```python
from build123d import *

# Parameters (mm, degrees)
ESQUISSE1_R             = 15
BOSS_EXTRU_1_DEPTH      = 20
ESQUISSE3_R             = 13.5
ENL_V_MAT_EXTRU_2_DEPTH = 19
ESQUISSE4_R             = 12.5
BOSS_EXTRU_2_DEPTH      = 1
ESQUISSE5_R             = 11
ENL_V_MAT_EXTRU_3_DEPTH = 2


with BuildPart() as part:
    # Esquisse1 → Boss.-Extru.1 (new body)
    with BuildSketch(Plane.XY):
        Circle(ESQUISSE1_R)
    extrude(amount=BOSS_EXTRU_1_DEPTH)

    # Esquisse3 → Enlèv. mat.-Extru.2 (cut)
    with BuildSketch(Plane(origin=(0, 0, 0), x_dir=(-1, 0, 0), z_dir=(0, 0, -1))):
        Circle(ESQUISSE3_R)
    extrude(amount=-ENL_V_MAT_EXTRU_2_DEPTH, mode=Mode.SUBTRACT)

    # Esquisse4 → Boss.-Extru.2 (add)
    with BuildSketch(Plane.XY.offset(20)):
        Circle(ESQUISSE4_R)
    extrude(amount=BOSS_EXTRU_2_DEPTH)

    # Esquisse5 → Enlèv. mat.-Extru.3 (cut)
    with BuildSketch(Plane.XY.offset(21)):
        Circle(ESQUISSE5_R)
    extrude(amount=-ENL_V_MAT_EXTRU_3_DEPTH, mode=Mode.SUBTRACT)


solid = part.part
```
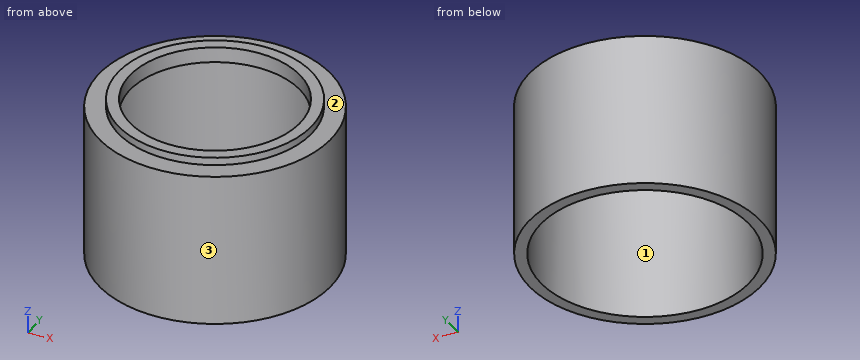
Check sheet for the modelled part. Datum: model origin and axes. Units: mm. Face numbers are marked on the shaded views. Coordinates: 2 decimals unless noted, no trailing zeros. Write each loop counter-clockwise with the first axis right and the second up, starting at its lowest first coordinate (ties: lowest second). Pieces come first, ordered by that corner, then holes. Notation, with made-up numbers: (55.5, -4) - (80.5, -4) arc R19 cw to (80.5, 23) - close; hole circle Ø10 at (-33.5, -27). An arc over 180 degrees is marked (long way). One line per question, with ' | ' between items.
Item 1: Thickness scan on line 1 (Y direction, x = 0, z = 20.1); line 2 (Y direction, x = 0, z = 11.75); line 3 (X direction, y = 4, z = 1.25). Record the ranges inside material, lowest first. Write a range as [from, to].
Determined:
line 1: y = [-12.5, -11], [11, 12.5] | line 2: y = [-15, -13.5], [13.5, 15] | line 3: x = [-14.46, -12.89], [12.89, 14.46]
Item 2: Gauge pin test, flat ends, axial feed: P1, Ø5, axis at x = 10.5, z = 17.5, coming from the +Y side; P2, Ø1, axis at x = -6.5, z = 15, coming from the +Y side; P3, Ø3, axis at x = -8, y = 5.5, coming from the +Z side; P4, Ø12, axis at y = -11, z = 18, coming from the -X side. Record the tip position at first contact, or that the pin passes through.
Determined:
P1: stops at y = 12.69 | P2: stops at y = 13.75 | P3: stops at z = 21 | P4: stops at x = -14.14
Item 3: Sectioned sample at C-C on z = 14.25. Record the boundary of the cut face in (x, y).
Determined:
outline: circle Ø30 at (0, 0); hole circle Ø27 at (0, 0)
Item 4: Sectioned sample at A-A on y = 0. Record the boundary of the cut face in (x, z), plus the area to 3 significant figures.
Determined:
outline: (-15, 0) - (-13.5, 0) - (-13.5, 19) - (-11, 19) - (-11, 21) - (-12.5, 21) - (-12.5, 20) - (-15, 20) - close; (11, 19) - (13.5, 19) - (13.5, 0) - (15, 0) - (15, 20) - (12.5, 20) - (12.5, 21) - (11, 21) - close | area: 68.0 mm2
Item 5: Mould release check, pull along Y, two halves, no side actions. Record for the marked faces 1, 2 and 3: pulls with the +Y half, pulls with the -Y half, needs draft (parallel to the pull), parting line crosses it, or undercut.
Determined:
face 1: undercut | face 2: needs draft | face 3: parting line crosses it
